Source: three-view drawing plus pictorial views. Frame: mm from the lowest corner of the part. Coordinates: 2 decimals unless noted, no trailing zeros. Write each loop counter-clockwise with the first axis right and the second up, starting at its lowest first coordinate (ties: lowest second). Pieces come first, ordered by that corner, then holes. Notation, with made-up numbers: (84.25, 6) -> (124.25, 6) arc R19 cw to (124.25, 29) -> close; hole circle Ø8 at (-14.75, 29). An arc over 180 degrees is marked (long way). One line per item, written item: value. Start each with the question number.
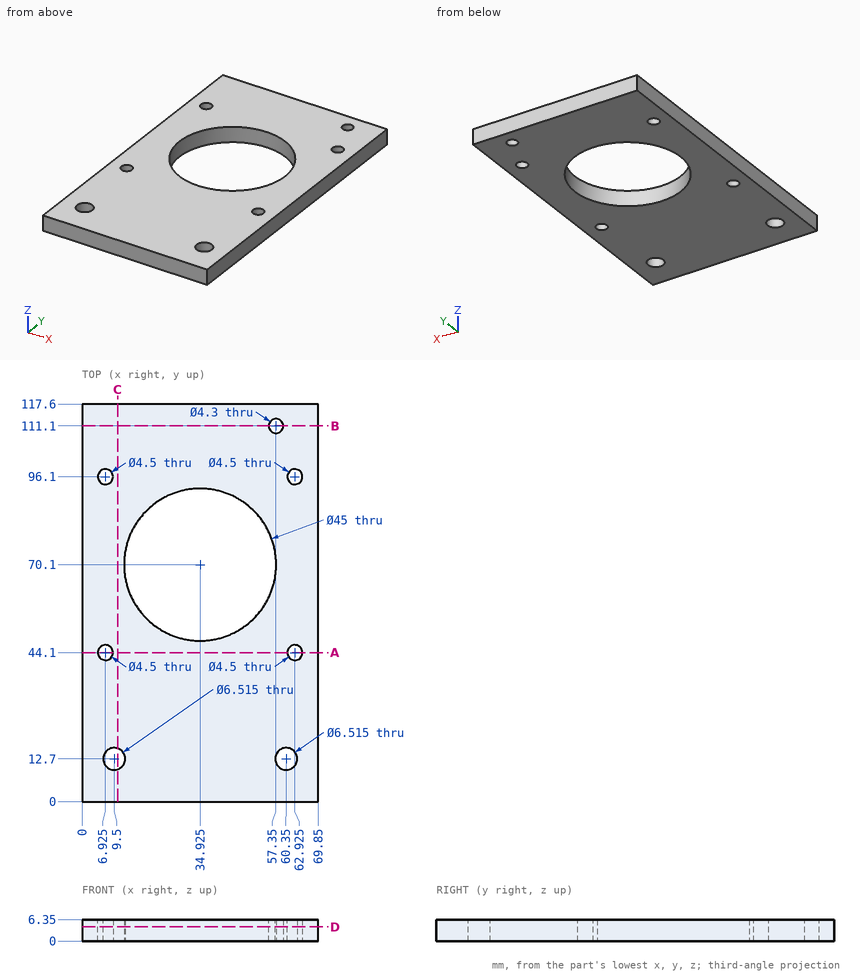
Q1. Cut plane A-A on y = 44.1. Output: boundary loops of the cut face in (x, z) (3 decimals), and give its area (3 significant figures).
Q2. Line query: L1, parallel to Y at x = 64.5, z = 4.25; L2, parallel to Y at x = 55.5, z = 1.5 (1 decimal); L3, parallel to Y at x = 47, z = 3.5 (1 decimal). Output: solid intervals per line, ascending. Write a range as from..to.
Q3. Cut plane D-D on z = 4.25. Count the separate pieces of the cut face and the enclosed holes in it, and give its area (3 significant figures).
Q4. Cut plane B-B on y = 111.1. Output: boundary loops of the cut face in (x, z).
Q5. First-contact query: P1, Ø6, axis at x = 60.35, y = 12.7, coming from the +Z side. Flat tip, straight axial feed; report the tip coordinate or a pass-through.
Q6. Cut plane C-C on x = 10.5. Output: boundary loops of the cut face in (y, z).
Solution:
1. outline: (0, 0) -> (4.675, 0) -> (4.675, 6.35) -> (0, 6.35) -> close; (9.175, 0) -> (60.675, 0) -> (60.675, 6.35) -> (9.175, 6.35) -> close; (65.175, 0) -> (69.85, 0) -> (69.85, 6.35) -> (65.175, 6.35) -> close
1. area: 386 mm²
2. L1: 0..42.49, 45.71..94.49, 97.71..117.6
2. L2: 0..61, 79.2..110, 112.2..117.6
2. L3: 0..51.1, 89.1..117.6
3. separate pieces: 1
3. enclosed holes: 8
3. area: 6,480 mm²
4. outline: (0, 0) -> (55.2, 0) -> (55.2, 6.35) -> (0, 6.35) -> close; (59.5, 0) -> (69.85, 0) -> (69.85, 6.35) -> (59.5, 6.35) -> close
5. P1: through
6. outline: (0, 0) -> (9.6, 0) -> (9.6, 6.35) -> (0, 6.35) -> close; (15.8, 0) -> (117.6, 0) -> (117.6, 6.35) -> (15.8, 6.35) -> close
